Verification items for the finished model (mm, model axes). A direction names the side the tool comes from. Give positions to 0.01 mm unless a question says otherwise; leave off trailing zeros. Order: outer loops, then holes, each group sorted by start corner. A loop starts at its lowest first (then second) coordinate and runs counter-clockwise, first axis right, second up. Notation, with made-up numbers: (13.25, 40.5) -> (25.25, 40.5) arc R31 cw to (25.25, 77.5) -> close; hole circle Ø9 at (-6, 8). An arc over 180 degrees is marked (long way). One line per question, with ' | ' between items. Start each with the question number.
Q1. Section check D-D on y = 35. Record the cut outline in (x, z), plus the area to 3 significant figures.
Q2. Mould release check, pull along Y, two halves, no side actions. Record for faces 5 (the flat face through (7, 7, 28.575)), 6 (the cylindrical face through (-1.494, 37.547, 16.701)), 7 (the cylindrical face through (-1.5, 2.8, 18.6)), 8 (the flat face through (30, 24.129, 16)): released by +Y, released by -Y, zero draft, split by the parting line, or undercut.
Q3. Access from +Z, -Z, +X, -X, +Y, -Y to the whole of each face (thin tool, end or side, straight path). Record for faces 1 (the flat face through (31.894, 18, 16)), 2 (the flat face through (6, 8, 3.175)), 3 (the flat face through (12, 12.37, 30)), 4 (the flat face through (0.144, 30, 16)).
Q4. Material ranges on probe 1 along X at (y, z) = (19.5, 14); probe 2 along Y at (x, z) = (5, 6.5); probe 3 along X at (y, z) = (-1, 3.5), recorded low to high. Write a range as [from, to].
Q5. Section check C-C on x = 8. Record the cut outline in (y, z) (3 decimals), plus the area to 3 significant figures.
Q6. Section check B-B on z = 30.5. Record the cut outline in (x, y), plus the area to 3 significant figures.
Q7. Section check A-A on y = 23.5. Record the cut outline in (x, z).
Q8. Go/stop test with flat-tipped pins: pin 1 (20.5 mm diameter, centred on x = 13, y = 5, fed in from -Z); pin 2 (2 mm diameter, centred on x = 9, z = 3.5, fed in from -Y); pin 3 (14.5 mm diameter, centred on x = 19.5, z = 16, fed in from +Y); pin 4 (12 mm diameter, centred on x = 10, z = 17, fed in from -Y). Record where each tip stops, or that it passes through.
from build123d import *

# Parameters (mm, degrees)
F1_DEPTH = 31.75
F3_DEPTH = 3.175
F5_DEPTH = 3.175
F7_D     = 5.5
F7_DEPTH = 3.0323066673


with BuildPart() as f1:
    # F0 (on Top) → F1 (new body)
    with BuildSketch(Plane.XY):
        Polygon((0.1436933327, 44.4485164799), (-3.0313066673, 44.4485164799), (-3.0313066673, -6.3514835201), (0.1436933327, -6.3514835201), (0.1436933327, 12.6985164799), (31.8936933327, 12.6985164799), (31.8936933327, 24.1285164799), (28.7186933327, 24.1285164799), (28.7186933327, 15.8735164799), (0.1436933327, 15.8735164799), align=None)
    extrude(amount=F1_DEPTH)

    # F2 (on Top) → F3 (join)
    with BuildSketch(Plane.XY):
        with BuildLine():
            ThreePointArc((0, -5.9709572233), (9.7535685251, 6.3565785033), (24.1138786077, 12.7504607663))
            Line((24.1138786077, 12.7504607663), (0, 12.7504607663))
            Line((0, 12.7504607663), (0, -5.9709572233))
        make_face()
    extrude(amount=F3_DEPTH)

    # F4 (on face) → F5 (join)
    with BuildSketch(Plane.XY.offset(31.75)):
        with BuildLine():
            ThreePointArc((0.1436933327, -6.0840700046), (9.8903219557, 6.066105621), (24.1341023211, 12.3699344695))
            Line((24.1341023211, 12.3699344695), (0.1436933327, 12.3699344695))
            Line((0.1436933327, 12.3699344695), (0.1436933327, -6.0840700046))
        make_face()
    extrude(amount=-F5_DEPTH)

    # F7 (through all, one way)
    with BuildSketch(Plane.YZ):
        with Locations((3.1735164799, 15.875), (34.9235164799, 15.875)):
            Circle(F7_D / 2)
    extrude(amount=-F7_DEPTH, mode=Mode.SUBTRACT)


solid = f1.part
Filled in:
1) outline: (-3.03, 0) -> (0.14, 0) -> (0.14, 31.75) -> (-3.03, 31.75) -> (-3.03, 18.62) -> (0, 18.62) -> (0, 13.13) -> (-3.03, 13.13) -> close | area: 84.1 mm²
2) face 5: zero draft | face 6: undercut | face 7: undercut | face 8: released by +Y
3) face 1: +Z, -Z, +X, +Y, -Y | face 2: +X, -Y | face 3: +Z, +X | face 4: +Z, -Z, +Y
4) probe 1: [-3.03, 0.14], [28.72, 31.89] | probe 2: [12.7, 15.87] | probe 3: [-3.03, 0.14]
5) outline: (4.496, 28.575) -> (12.37, 28.575) -> (12.37, 31.75) -> (4.496, 31.75) -> close; (4.895, 0) -> (15.874, 0) -> (15.874, 31.75) -> (12.699, 31.75) -> (12.699, 3.175) -> (4.895, 3.175) -> close | area: 151 mm²
6) outline: (-3.03, -6.35) -> (0.14, -6.35) -> (0.14, -6.08) arc R32.89 cw to (24.13, 12.37) -> (0.14, 12.37) -> (0.14, 12.7) -> (31.89, 12.7) -> (31.89, 24.13) -> (28.72, 24.13) -> (28.72, 15.87) -> (0.14, 15.87) -> (0.14, 44.45) -> (-3.03, 44.45) -> close | area: 434 mm²
7) outline: (-3.03, 0) -> (0.14, 0) -> (0.14, 31.75) -> (-3.03, 31.75) -> close; (28.72, 0) -> (31.89, 0) -> (31.89, 31.75) -> (28.72, 31.75) -> close
8) pin 1: z = 0 | pin 2: y = 4.94 | pin 3: y = 15.87 | pin 4: y = 12.7
